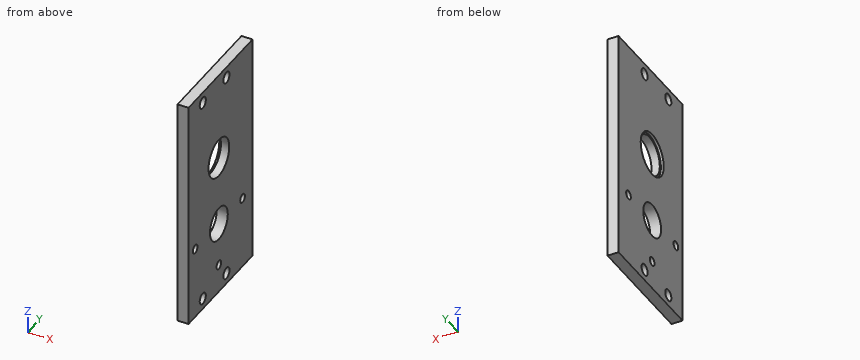
```python
from build123d import *

# Parameters (mm, degrees)
SKETCH1_W           = 133.35
SKETCH1_H           = 68.58
SKETCH1_R           = 11.1125
SKETCH1_R_2         = 9.5504
SKETCH1_R_3         = 2.4892
SKETCH1_R_4         = 3.2639
BOSS_EXTRUDE1_DEPTH = 6.35
SKETCH2_R           = 12.3063
CUT_EXTRUDE1_DEPTH  = 1.5875


with BuildPart() as part:
    # Sketch1 → Boss-Extrude1 (new body)
    with BuildSketch(Plane(origin=(0, 0, 0), x_dir=(0, 0, -1), z_dir=(1, 0, 0))):
        with Locations((15.875, 1.778)):
            Rectangle(SKETCH1_W, SKETCH1_H)
        Circle(SKETCH1_R, mode=Mode.SUBTRACT)
        with Locations((40.6654, 0)):
            Circle(SKETCH1_R_2, mode=Mode.SUBTRACT)
        with Locations((40.6654, 25.4)):
            Circle(SKETCH1_R_3, mode=Mode.SUBTRACT)
        with Locations((40.6654, -25.4)):
            Circle(SKETCH1_R_3, mode=Mode.SUBTRACT)
        with Locations((66.0654, 0)):
            Circle(SKETCH1_R_3, mode=Mode.SUBTRACT)
        with Locations((76.2, -17.272)):
            Circle(SKETCH1_R_4, mode=Mode.SUBTRACT)
        with Locations((76.2, 8.128)):
            Circle(SKETCH1_R_4, mode=Mode.SUBTRACT)
        with Locations((-44.45, 8.128)):
            Circle(SKETCH1_R_4, mode=Mode.SUBTRACT)
        with Locations((-44.45, -17.272)):
            Circle(SKETCH1_R_4, mode=Mode.SUBTRACT)
    extrude(amount=BOSS_EXTRUDE1_DEPTH)

    # Sketch2 → Cut-Extrude1 (cut)
    with BuildSketch(Plane.ZY):
        Circle(SKETCH2_R)
    extrude(amount=-CUT_EXTRUDE1_DEPTH, mode=Mode.SUBTRACT)


solid = part.part
```
Design review of the part built by this model. Coordinates are the model's own, in mm. Coordinates: 2 decimals unless noted, no trailing zeros. Write each loop counter-clockwise with the first axis right and the second up, starting at its lowest first coordinate (ties: lowest second). Pieces come first, ordered by that corner, then holes.
1) Add section C-C (z = 0). Write out the cut boundary in (x, y), plus the area to 3 significant figures.
2) Insertion check: pin 1 (10 mm diameter, centred on y = -18, z = -68, fed in from -X). The pin has a flat end and moves straight along its axis. Give the tip position at first contact, or say it passes through.
3) Add section A-A (z = -76.2). Write out the cut boundary in (x, y).
4) Add section B-B (y = 25.4). Write out the cut boundary in (x, z), plus the area to 3 significant figures.
5) To check wall thickness, follow L1, parallel to Y at x = 1.5, z = 44.45; L2, parallel to Z at x = 2.5, y = -4.5; L3, parallel to Z at x = 1.5, y = 11. State the ranges of each line that lie inside material, in increasing order.
6) Add section D-D (x = 3). State how many separate pieces and enclosed holes the cut face has, plus the area to 3 significant figures.
Check result:
1. outline: (0, -32.51) - (6.35, -32.51) - (6.35, -11.11) - (1.59, -11.11) - (1.59, -12.31) - (0, -12.31) - close; (0, 12.31) - (1.59, 12.31) - (1.59, 11.11) - (6.35, 11.11) - (6.35, 36.07) - (0, 36.07) - close
1. area: 291 mm2
2. pin 1: stops at x = 0
3. outline: (0, -32.51) - (6.35, -32.51) - (6.35, -20.54) - (0, -20.54) - close; (0, -14.01) - (6.35, -14.01) - (6.35, 4.86) - (0, 4.86) - close; (0, 11.39) - (6.35, 11.39) - (6.35, 36.07) - (0, 36.07) - close
4. outline: (0, -82.55) - (6.35, -82.55) - (6.35, -43.15) - (0, -43.15) - close; (0, -38.18) - (6.35, -38.18) - (6.35, 50.8) - (0, 50.8) - close
4. area: 815 mm2
5. L1: y = -32.51 to -20.54, -14.01 to 4.86, 11.39 to 36.07
5. L2: z = -82.55 to -49.09, -32.24 to -10.16, 10.16 to 50.8
5. L3: z = -82.55 to -77.75, -74.65 to -5.52, 5.52 to 42.9, 46 to 50.8
6. separate pieces: 1
6. enclosed holes: 9
6. area: 8,280 mm2
